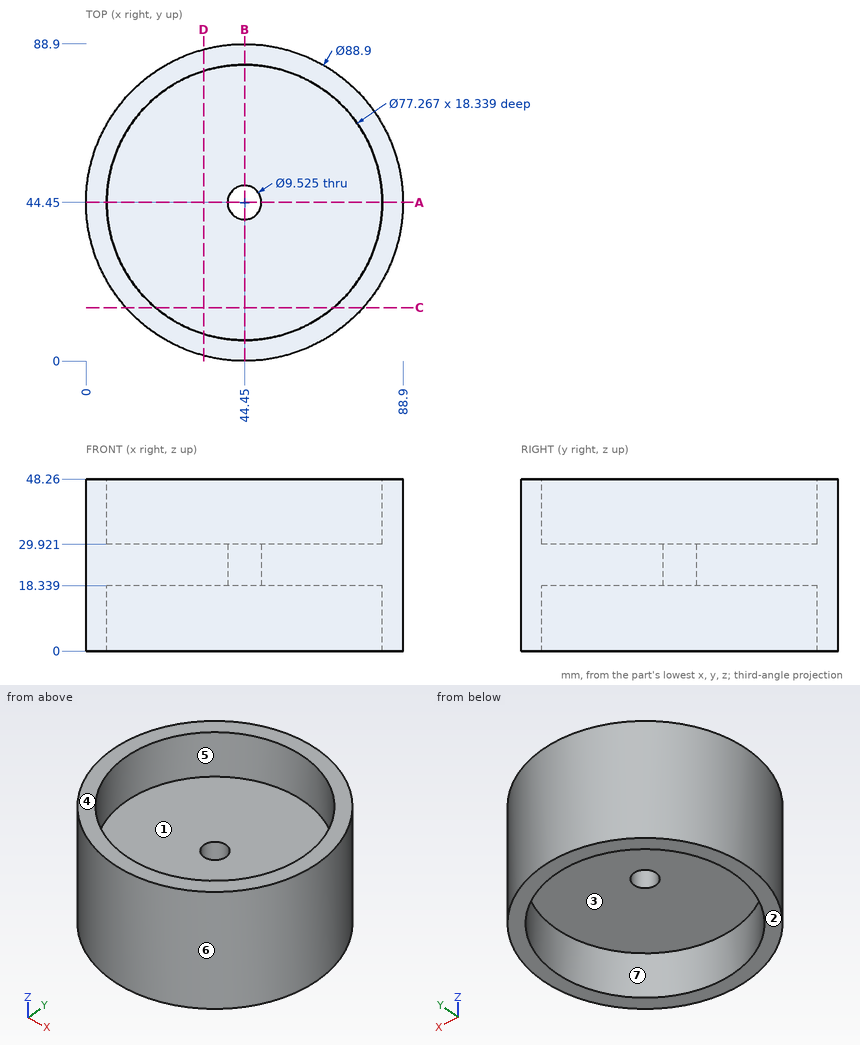
Could you check a few things on this drawing? It's one solid part, dimensions in mm from its lowest x, y, z. A direction names the side the tool comes from. Coordinates: 2 decimals unless noted, no trailing zeros. Loops run counter-clockwise (first coordinate to the right, second up) from the corner with the lowest first, then second, coordinate; pieces in that order, holes last.
1. Imagine slicing it at D-D (x = 33). Please give me the cut outline in (y, z), and give its area (3 significant figures).
2. Imagine slicing it at C-C (y = 15). Please give me the cut outline in (x, z) (1 decimal).
3. We'd pull the mould along X, two halves only. Please class the marked faces 4, 5, 6 and 7: released by +X, released by -X, zero draft, split by the parting line, or undercut.
4. For P1, Ø2, axis at x = 26.5, y = 35.5, coming from the +Z side; P2, Ø4, axis at x = 56, z = 41, coming from the -Y side; P3, Ø1.5, axis at y = 14.5, z = 11, coming from the +X side, each with a flat end and sliding along its axis, tell me the tip position at first contact or that it passes through.
5. For the marked faces 1, 2 and 3, which set-ups out of +Z, -Z, +X, -X, +Y, -Y let a thin tool reach every point of the face, with its end or its side?
6. I need wall thicknesses on L1, parallel to X at y = 44.45, z = 14.75; L2, parallel to Y at x = 44, z = 23. Which ranges of each line are inside material? Lowest first, please.
7. Imagine slicing it at A-A (y = 44.45). Please give me the cut outline in (x, z), and give its area (3 significant figures).
Computed values:
1. outline: (1.5, 0) - (7.55, 0) - (7.55, 18.34) - (81.35, 18.34) - (81.35, 0) - (87.4, 0) - (87.4, 48.26) - (81.35, 48.26) - (81.35, 29.92) - (7.55, 29.92) - (7.55, 48.26) - (1.5, 48.26) - close
1. area: 1,440 mm2
2. outline: (11.2, 0) - (19.4, 0) - (19.4, 18.3) - (69.5, 18.3) - (69.5, 0) - (77.7, 0) - (77.7, 48.3) - (69.5, 48.3) - (69.5, 29.9) - (19.4, 29.9) - (19.4, 48.3) - (11.2, 48.3) - close
3. face 4: zero draft
3. face 5: undercut
3. face 6: split by the parting line
3. face 7: undercut
4. P1: stops at z = 29.92
4. P2: stops at y = 1.04
4. P3: stops at x = 77.96
5. face 1: +Z
5. face 2: -Z, +X, -X, +Y, -Y
5. face 3: -Z
6. L1: x = 0 to 5.82, 83.08 to 88.9
6. L2: y = 0 to 39.71, 49.19 to 88.9
7. outline: (0, 0) - (5.82, 0) - (5.82, 18.34) - (39.69, 18.34) - (39.69, 29.92) - (5.82, 29.92) - (5.82, 48.26) - (0, 48.26) - close; (49.21, 18.34) - (83.08, 18.34) - (83.08, 0) - (88.9, 0) - (88.9, 48.26) - (83.08, 48.26) - (83.08, 29.92) - (49.21, 29.92) - close
7. area: 1,350 mm2
